Source: three-view drawing plus pictorial views. Frame: mm from the lowest corner of the part. Round coordinates to 2 decimals unless told otherwise and drop trailing zeros. Loops run counter-clockwise (first coordinate to the right, second up) from the corner with the lowest first, then second, coordinate; pieces in that order, holes last. Notation, with made-up numbers: (41.25, 67) -> (47.25, 67) arc R15 ccw to (47.25, 71) -> close; hole circle Ø9 at (36.5, 15.25). An arc over 180 degrees is marked (long way). One line per question, with ' | ' between items. Start each with the question number.
Q1. Cut plane C-C on x = 46.5. Return loops of the section in (y, z), and give its area (3 significant figures).
Q2. Cut plane A-A on z = 42.4. Return loops of the section in (x, y), and give its area (3 significant figures).
Q3. Cut plane B-B on y = 0.7. State how many separate pieces and enclosed holes the cut face has, and give its area (3 significant figures).
Q4. Contact query for flat-ended pins moving along their axis: P1, Ø2.5, axis at x = 20.93, z = 83.66, coming from the -Y side; P2, Ø1, axis at y = 1.5, z = 10.5, coming from the +X side; P3, Ø3.5, axis at x = 33.69, z = 62.4, coming from the -Y side (1 decimal); P4, Ø0.6, axis at x = 47, y = 1, coming from the +Z side. Output: stop coordinate, or through.
Q5. Cut plane D-D on z = 10. Return loops of the section in (x, y).
Q6. Material intervals for L1, parallel to X at y = 1.6, z = 62.4; L2, parallel to X at y = 1.2, z = 15 (1 decimal); L3, parallel to X at y = 0.2, z = 5, sorted ascending.
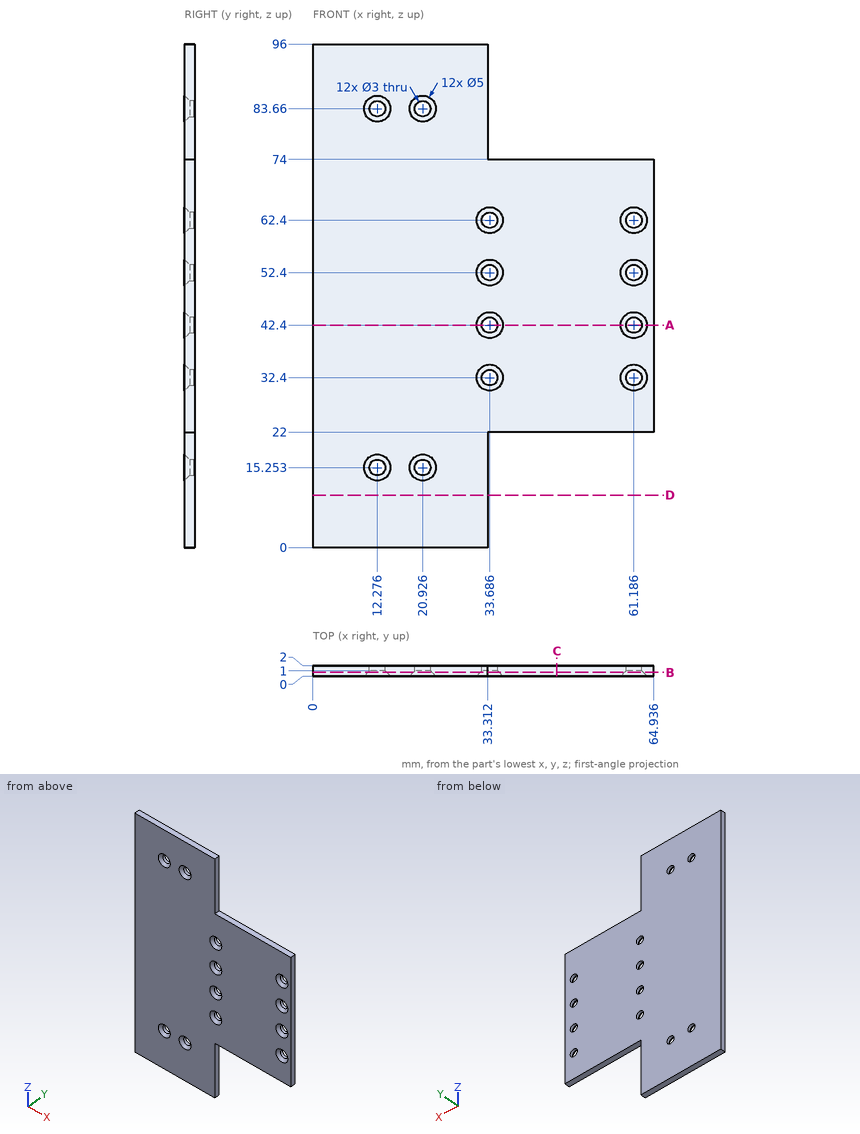
Results:
1) outline: (0, 22) -> (2, 22) -> (2, 74) -> (0, 74) -> close | area: 104 mm^2
2) outline: (0, 0) -> (31.19, 0) -> (32.19, 1) -> (32.19, 2) -> (0, 2) -> close; (35.19, 1) -> (36.19, 0) -> (58.69, 0) -> (59.69, 1) -> (59.69, 2) -> (35.19, 2) -> close; (62.69, 1) -> (63.69, 0) -> (64.94, 0) -> (64.94, 2) -> (62.69, 2) -> close | area: 116 mm^2
3) separate pieces: 1 | enclosed holes: 12 | area: 4,720 mm^2
4) P1: through | P2: x = 33.31 | P3: y = 0.7 | P4: z = 74
5) outline: (0, 0) -> (33.31, 0) -> (33.31, 2) -> (0, 2) -> close
6) L1: 0 to 32.19, 35.19 to 59.69, 62.69 to 64.94 | L2: 0 to 10.8, 13.8 to 19.4, 22.4 to 33.3 | L3: 0 to 33.31
